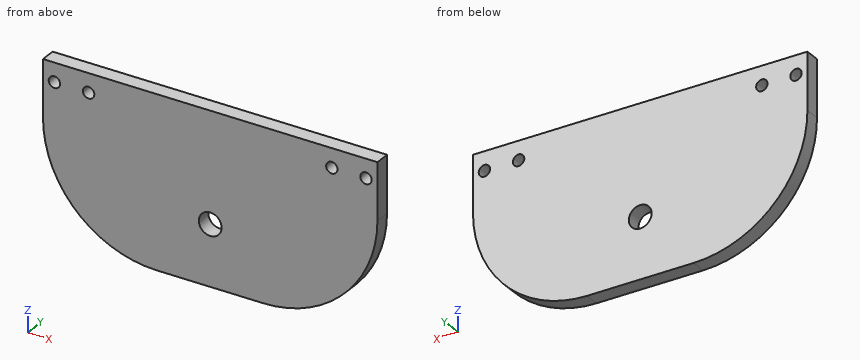
```python
from build123d import *

# Parameters (mm, degrees)
SKETCH_1_W          = 88
SKETCH_1_H          = 45
EXTRUDE_1_DEPTH     = 4
SKETCH_2_R          = 3
CUT_EXTRUDE_1_DEPTH = 4
SKETCH_3_R          = 1.5
CUT_EXTRUDE_2_DEPTH = 50.580742229
FILLET_1_R          = 30


with BuildPart() as part:
    # 草图1 → 凸台-拉伸1 (new body)
    with BuildSketch(Plane(origin=(0, 0, 0), x_dir=(1, 0, 0), z_dir=(0, 1, 0))):
        Rectangle(SKETCH_1_W, SKETCH_1_H)
    extrude(amount=EXTRUDE_1_DEPTH)

    # 草图2 → 切除-拉伸1 (cut)
    with BuildSketch(Plane(origin=(0, 4, 0), x_dir=(1, 0, 0), z_dir=(0, 1, 0))):
        with Locations(Location((0, 6.5, 0), (0, 0, 270))):
            Circle(SKETCH_2_R)
    extrude(amount=-CUT_EXTRUDE_1_DEPTH, mode=Mode.SUBTRACT)

    # 草图3 → 切除-拉伸2 (cut, through all)
    with BuildSketch(Plane(origin=(0, 4, 0), x_dir=(1, 0, 0), z_dir=(0, 1, 0))):
        with Locations(Location((-41, -17.5, 0), (0, 0, 270))):
            Circle(SKETCH_3_R)
        with Locations(Location((-32, -17.5, 0), (0, 0, 90))):
            Circle(SKETCH_3_R)
        with Locations(Location((32, -17.5, 0), (0, 0, 270))):
            Circle(SKETCH_3_R)
        with Locations(Location((41, -17.5, 0), (0, 0, 90))):
            Circle(SKETCH_3_R)
    extrude(amount=-CUT_EXTRUDE_2_DEPTH, mode=Mode.SUBTRACT)

    # 圆角1
    fillet_1_edges = [part.edges().sort_by_distance(p)[0] for p in [
        (-44, 2, -22.5),
        (44, 2, -22.5),
    ]]
    fillet(fillet_1_edges, radius=FILLET_1_R)


solid = part.part
```
Verification items for the finished model (mm, model axes). Round coordinates to 2 decimals unless told otherwise and drop trailing zeros. Write each loop counter-clockwise with the first axis right and the second up, starting at its lowest first coordinate (ties: lowest second). Pieces come first, ordered by that corner, then holes.
1. Section check A-A on x = 32. Enter the section's corners in (y, z), plus the area to 3 significant figures.
2. Gauge pin test, flat ends, axial feed: P1, Ø5, axis at x = -41, z = 17.5, coming from the -Y side; P2, Ø5.5, axis at x = 0, z = -6.5, coming from the +Y side; P3, Ø1.5, axis at y = 2, z = -3, coming from the +X side. Record the tip position at first contact, or that the pin passes through.
3. Scan lines: L1, parallel to X at y = 2, z = 17.5; L2, parallel to X at y = 0.4, z = 18; L3, parallel to X at y = 2.95, z = -6.5. Record each from-to range of solid material in increasing order.
4. Section check C-C on z = -6.5. Enter the section's corners in (x, y), plus the area to 3 significant figures.
5. Section check B-B on y = 1.25. Enter the section's corners in (x, z).
6. Section check D-D on x = -26. Enter the section's corners in (y, z).
Answer:
1. outline: (0, -16.5) - (4, -16.5) - (4, 16) - (0, 16) - close; (0, 19) - (4, 19) - (4, 22.5) - (0, 22.5) - close
1. area: 144 mm2
2. P1: stops at y = 0
2. P2: passes through
2. P3: stops at x = 42.37
3. L1: x = -44 to -42.5, -39.5 to -33.5, -30.5 to 30.5, 33.5 to 39.5, 42.5 to 44
3. L2: x = -44 to -42.41, -39.59 to -33.41, -30.59 to 30.59, 33.41 to 39.59, 42.41 to 44
3. L3: x = -40.53 to -3, 3 to 40.53
4. outline: (-40.53, 0) - (-3, 0) - (-3, 4) - (-40.53, 4) - close; (3, 0) - (40.53, 0) - (40.53, 4) - (3, 4) - close
4. area: 300 mm2
5. outline: (-44, 7.5) arc R30 ccw to (-14, -22.5) - (14, -22.5) arc R30 ccw to (44, 7.5) - (44, 22.5) - (-44, 22.5) - close; hole circle Ø3 at (-41, 17.5); hole circle Ø3 at (-32, 17.5); hole circle Ø6 at (0, -6.5); hole circle Ø3 at (32, 17.5); hole circle Ø3 at (41, 17.5)
6. outline: (0, -20) - (4, -20) - (4, 22.5) - (0, 22.5) - close
